The model under review builds one solid part; all positions refer to its coordinate system, in mm. A direction names the side the tool comes from. Round coordinates to 2 decimals unless told otherwise and drop trailing zeros. Write each loop counter-clockwise with the first axis right and the second up, starting at its lowest first coordinate (ties: lowest second). Pieces come first, ordered by that corner, then holes. Notation, with made-up numbers: (65, -31) -> (69, -31) arc R14 cw to (69, -20) -> close; hole circle Ø4 at (38.25, 52.25). An arc over 180 degrees is marked (long way). Use CSV: the item, a comma, the result in double quotes. Start each with the question number.
1) For pin 1 Ø3 at (y, z) = (2, 57.5) entering from +X; pin 2 Ø3 at (x, z) = (0.5, 31) entering from +Y; pin 3 Ø11.5 at (y, z) = (0.5, 42.5) entering from -X; pin 4 Ø8 at (x, y) = (8, 4) entering from +Z, all flat-tipped, find the tip position at first contact; note any pin that passes through.
2) Take a section at A-A, the plane z = 17. Give the boundary of the cut face in (x, y), then the cut area to 3 significant figures.
3) Take a section at C-C, the plane x = 2.25. Give the boundary of the cut face in (y, z), then the cut area to 3 significant figures.
4) Take a section at B-B, the plane y = 0. Give the boundary of the cut face in (x, z).
5) Wall thickness on probe 1 along Y at (x, z) = (-2, 83); probe 2 along X at (y, z) = (-6.75, 27): over which ranges is each line inside the solid? List them lowest first. Write a range as [from, to].
6) Take a section at D-D, the plane y = -8.75. Give the boundary of the cut face in (x, z), then the cut area to 3 significant figures.
7) Machinability: for faces 4 (the face through (11.923, 3.755, 1.479)), 5 (the face through (4.314, -7.613, -7.642)), 6 (the face through (5.25, 0, 47)), which of the approach directions +Z, -Z, +X, -X, +Y, -Y give a long, thin tool a straight path to every point of the face, cutting with its end or side? Answer none if there is none.
8) Mouldability with a two-part tool opening along X and no side actions: class faces 1 (the face through (7.5, 0, 48)), 2 (the face through (-8.75, 0, -8)), 3 (the face through (-7.5, 0, 48)) as released by +X, released by -X, zero draft, split by the parting line, or undercut.
from build123d import *

# Parameters (mm, degrees)
F0_W     = 15
F0_H     = 15
F0_W_2   = 10.5
F0_H_2   = 10.5
F1_DEPTH = 95
F2_R     = 15
F3_DEPTH = 15.5
F4_R     = 12.5
F4_W     = 15
F4_H     = 15
F5_DEPTH = 3


with BuildPart() as f1:
    # F0 (on Top) → F1 (new body)
    with BuildSketch(Plane.XY):
        Rectangle(F0_W, F0_H)
        Rectangle(F0_W_2, F0_H_2, mode=Mode.SUBTRACT)
    extrude(amount=F1_DEPTH)

    # F2 (on face) → F3 (join)
    with BuildSketch(Plane(origin=(0, 0, 0), x_dir=(1, 0, 0), z_dir=(0, 0, -1))):
        Circle(F2_R)
        Polygon((0, -10.10363), (-8.75, -5.051815), (-8.75, 5.051815), (0, 10.10363), (8.75, 5.051815), (8.75, -5.051815), align=None, mode=Mode.SUBTRACT)
    extrude(amount=F3_DEPTH)

    # F4 (on face) → F5 (join)
    with BuildSketch(Plane.XY):
        Circle(F4_R)
        Rectangle(F4_W, F4_H, mode=Mode.SUBTRACT)
    extrude(amount=F5_DEPTH)


solid = f1.part
Values found:
1,pin 1,"x = 7.5"
1,pin 2,"y = 7.5"
1,pin 3,"x = -7.5"
1,pin 4,"z = 95"
2,outline,"(-7.5, -7.5) -> (7.5, -7.5) -> (7.5, 7.5) -> (-7.5, 7.5) -> close; hole (-5.25, -5.25) -> (5.25, -5.25) -> (5.25, 5.25) -> (-5.25, 5.25) -> close"
2,area,"115 mm²"
3,outline,"(-14.83, -15.5) -> (-8.8, -15.5) -> (-8.8, 0) -> (-5.25, 0) -> (-5.25, 95) -> (-7.5, 95) -> (-7.5, 3) -> (-12.3, 3) -> (-12.3, 0) -> (-14.83, 0) -> close; (5.25, 0) -> (8.8, 0) -> (8.8, -15.5) -> (14.83, -15.5) -> (14.83, 0) -> (12.3, 0) -> (12.3, 3) -> (7.5, 3) -> (7.5, 95) -> (5.25, 95) -> close"
3,area,"643 mm²"
4,outline,"(-15, -15.5) -> (-8.75, -15.5) -> (-8.75, 0) -> (-5.25, 0) -> (-5.25, 95) -> (-7.5, 95) -> (-7.5, 3) -> (-12.5, 3) -> (-12.5, 0) -> (-15, 0) -> close; (5.25, 0) -> (8.75, 0) -> (8.75, -15.5) -> (15, -15.5) -> (15, 0) -> (12.5, 0) -> (12.5, 3) -> (7.5, 3) -> (7.5, 95) -> (5.25, 95) -> close"
5,probe 1,"[-7.5, -5.25], [5.25, 7.5]"
5,probe 2,"[-7.5, 7.5]"
6,outline,"(-12.18, -15.5) -> (-2.34, -15.5) -> (-2.34, 0) -> (2.34, 0) -> (2.34, -15.5) -> (12.18, -15.5) -> (12.18, 0) -> (8.93, 0) -> (8.93, 3) -> (-8.93, 3) -> (-8.93, 0) -> (-12.18, 0) -> close"
6,area,"359 mm²"
7,face 4,"+Z"
7,face 5,"-Z"
7,face 6,"+Z, -Z"
8,face 1,"released by +X"
8,face 2,"undercut"
8,face 3,"released by -X"
